The listing builds one solid part. Answer for the finished solid, in the listing's coordinates (mm). Coordinates: 2 decimals unless noted, no trailing zeros. Loops run counter-clockwise (first coordinate to the right, second up) from the corner with the lowest first, then second, coordinate; pieces in that order, holes last. Notation, with made-up numbers: (58.5, 28.25) - (66.5, 28.25) arc R33 cw to (66.5, 56.25) - close; hole circle Ø4 at (-8.75, 2). An arc over 180 degrees is marked (long way). Return JSON: item names as keys, results as strings. Group by question number.
1. Section C-C (y = 28) is taken. Write down the section's boundary in (x, z).
2. Section B-B (x = 18) is taken. Write down the section's boundary in (y, z), and give its area (3 significant figures).
3. Find the intervals of material crossed by line 1 along X through (y, z) = (8, -0.3); line 2 along X through (y, z) = (-9, -0.05); line 3 along X through (y, z) = (8.5, -0.1), in increasing order.
4. This flat-tipped pin is pushed along its axis until it touches: P1, Ø4.5, axis at x = 0, y = 28.5, coming from the -Z side. Where does it stop, or does it pass through?
5. Section A-A (x = 0) is taken. Write down the section's boundary in (y, z).
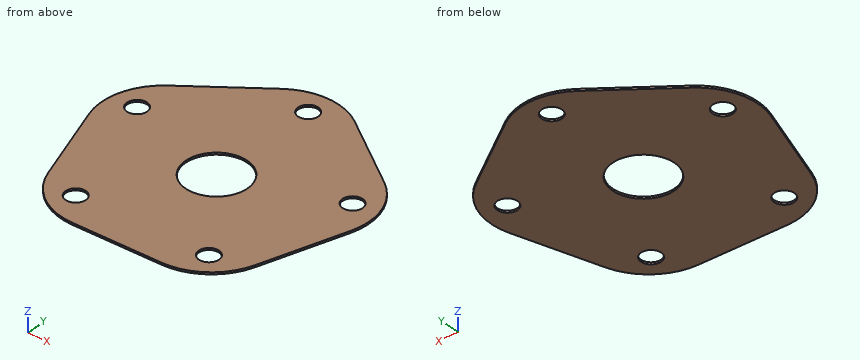
Solid Edge part; units mm, degrees
sketch "Sketch1" plane through (0, 0, 0) normal (0, 0, -1) x (-1, 0, 0)
  line L0 (-9.1636, 31.6216) -> (-27.2423, 18.4866)
  arc A0 (-27.2423, 18.4866) -> (-32.9056, 1.0566) centre (-18.0788, 5.8742) ccw
  line L1 (-32.9056, 1.0566) -> (-26.0002, -20.1962)
  arc A1 (-26.0002, -20.1962) -> (-11.1732, -30.9686) centre (-11.1732, -15.3786) ccw
  line L2 (-11.1732, -30.9686) -> (11.1732, -30.9686)
  arc A2 (26.0002, -20.1962) -> (11.1732, -30.9686) centre (11.1732, -15.3786) cw
  line L3 (26.0002, -20.1962) -> (32.9056, 1.0565)
  arc A3 (32.9056, 1.0565) -> (27.2422, 18.4867) centre (18.0786, 5.8741) ccw
  line L4 (27.2422, 18.4867) -> (9.1636, 31.6216)
  arc A4 (9.1636, 31.6216) -> (-9.1636, 31.6216) centre (0, 19.009) ccw
extrude "Protrusion1" add sketch "Sketch1" along normal blind 0.5
hole "Furat_1" at (27.1051, 8.807, -0.5) direction (0, 0, 1) diameter 5.1 end through all
pattern_circular "MintaElőfordulás_1" count 5 over 360 about axis through (0, 0, -0.5) along (0, 0, 1) of "Furat_1"
sketch "Sketch2" plane through (0, 1.8152, -0.5) normal (0, 0, -1) x (-0.309017, 0.9510565, 0)
  circle A0 centre (-1.7263, -0.5609) radius 7.8
extrude "Kivágás_1" cut sketch "Sketch2" against normal blind 32.365
properties material "Szilikon"
The answers:
{
 "1": {"outline": "(-14.15, -0.5) - (-2.5, -0.5) - (-2.5, 0) - (-14.15, 0) - close; (2.5, -0.5) - (14.15, -0.5) - (14.15, 0) - (2.5, 0) - close"},
 "2": {"outline": "(-29.39, -0.5) - (-25.28, -0.5) - (-25.28, 0) - (-29.39, 0) - close; (-20.83, -0.5) - (25.2, -0.5) - (25.2, 0) - (-20.83, 0) - close", "area": "25.1 mm2"},
 "3": {"line 1": "x = -33.52 to -29.52, -24.69 to 24.69, 29.52 to 33.52", "line 2": "x = -29.64 to 29.64", "line 3": "x = -33.45 to -29.64, -24.57 to 24.57, 29.64 to 33.45"},
 "4": {"P1": "passes through"},
 "5": {"outline": "(-30.97, -0.5) - (-7.8, -0.5) - (-7.8, 0) - (-30.97, 0) - close; (7.8, -0.5) - (25.95, -0.5) - (25.95, 0) - (7.8, 0) - close; (31.05, -0.5) - (34.6, -0.5) - (34.6, 0) - (31.05, 0) - close"}
}
